Read the model definition and answer for the solid it produces. Units are mm, in the model's axes. Round coordinates to 2 decimals unless told otherwise and drop trailing zeros. Write each loop counter-clockwise with the first axis right and the second up, starting at its lowest first coordinate (ties: lowest second). Pieces come first, ordered by that corner, then holes. Notation, with made-up numbers: (73.5, 47) - (111.5, 47) arc R28 ccw to (111.5, 85) - close; hole circle Ø11 at (-25.75, 30.25). An arc over 180 degrees is marked (long way). One line per item, written item: value. Start each with the question number.
(1) Find the intervals of material crossed by L1, parallel to Y at x = 0, z = -9.5; L2, parallel to X at y = -207.5, z = -8.25; L3, parallel to X at y = -177, z = -11.5, in increasing order.
(2) A flat-ended cylindrical pin translates along its axis: pin 1 Ø3 at (x, z) = (137.5, -6.5) entering from -Y. Find the tip coordinate at first contact, or state that the pin passes through.
(3) A cutting plane is placed at A-A, the plane x = 0. Determine the outline of the cut face in (y, z) (3 decimals), plus the area to 3 significant figures.
(4) A cutting plane is placed at C-C, the plane z = -8.25. Determine the outline of the cut face in (x, y), plus the area to 3 significant figures.
(5) A cutting plane is placed at B-B, the plane y = 0. Determine the outline of the cut face in (x, z) (3 decimals).
(6) A cutting plane is placed at D-D, the plane x = 78. Determine the outline of the cut face in (y, z) (3 decimals), plus the area to 3 significant figures.
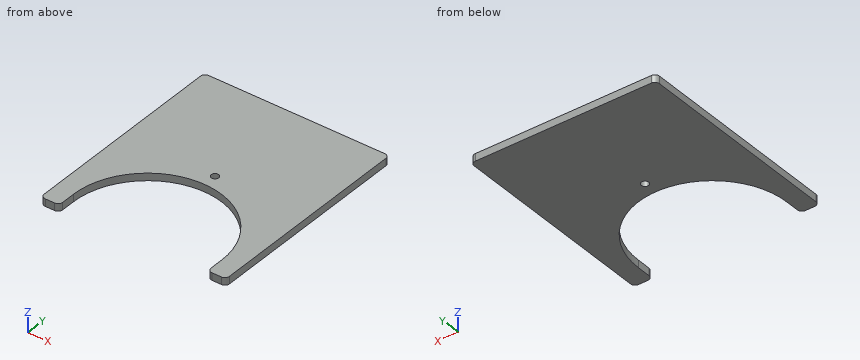
from build123d import *

# Parameters (mm, degrees)
SKETCH1_W           = 400
SKETCH1_H           = 460
BOSS_EXTRUDE1_DEPTH = 15.875
CUT_EXTRUDE1_DEPTH  = 306.208151308
FILLET1_R           = 10
SKETCH3_R           = 8
CUT_EXTRUDE2_DEPTH  = 306.208151308


with BuildPart() as part:
    # Sketch1 → Boss-Extrude1 (new body)
    with BuildSketch(Plane.XY):
        Rectangle(SKETCH1_W, SKETCH1_H)
    extrude(amount=-BOSS_EXTRUDE1_DEPTH)

    # Sketch2 → Cut-Extrude1 (cut, through all)
    with BuildSketch(Plane.XY):
        with BuildLine():
            Line((160, -230), (160, -190))
            ThreePointArc((160, -190), (0, -30), (-160, -190))
            Line((-160, -190), (-160, -230))
            Line((-160, -230), (160, -230))
        make_face()
    extrude(amount=-CUT_EXTRUDE1_DEPTH, mode=Mode.SUBTRACT)

    # Fillet1
    fillet1_edges = [part.edges().sort_by_distance(p)[0] for p in [
        (160, -230, -7.9375),
        (-160, -230, -7.9375),
        (200, -230, -7.9375),
        (-200, -230, -7.9375),
        (-200, 230, -7.9375),
        (200, 230, -7.9375),
    ]]
    fillet(fillet1_edges, radius=FILLET1_R)

    # Sketch3 → Cut-Extrude2 (cut, through all)
    with BuildSketch(Plane.XY):
        Circle(SKETCH3_R)
    extrude(amount=-CUT_EXTRUDE2_DEPTH, mode=Mode.SUBTRACT)


solid = part.part
Here are the results:
1. L1: -30 to -8, 8 to 230
1. L2: -200 to -160, 160 to 200
1. L3: -200 to -159.47, 159.47 to 200
2. pin 1: y = -110.76
3. outline: (-30, -15.875) - (-8, -15.875) - (-8, 0) - (-30, 0) - close; (8, -15.875) - (230, -15.875) - (230, 0) - (8, 0) - close
3. area: 3,870 mm²
4. outline: (-200, -220) arc R10 ccw to (-190, -230) - (-170, -230) arc R10 ccw to (-160, -220) - (-160, -190) arc R160 cw to (160, -190) - (160, -220) arc R10 ccw to (170, -230) - (190, -230) arc R10 ccw to (200, -220) - (200, 220) arc R10 ccw to (190, 230) - (-190, 230) arc R10 ccw to (-200, 220) - close; hole circle Ø16 at (0, 0)
4. area: 131,000 mm²
5. outline: (-200, -15.875) - (-8, -15.875) - (-8, 0) - (-200, 0) - close; (8, -15.875) - (200, -15.875) - (200, 0) - (8, 0) - close
6. outline: (-50.3, -15.875) - (230, -15.875) - (230, 0) - (-50.3, 0) - close
6. area: 4,450 mm²
